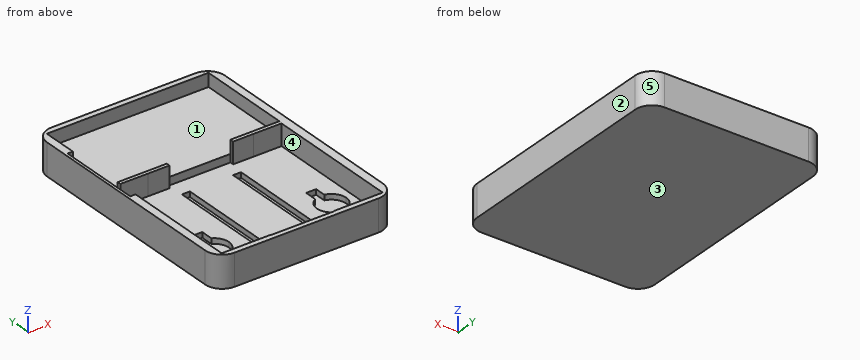
```python
from build123d import *

# Parameters (mm, degrees)
F1_DEPTH = 12
F3_DEPTH = 5
F2_W     = 24
F2_H     = 53
F5_DEPTH = 8
F6_DEPTH = 10
F7_W     = 3
F7_H     = 40
F8_DEPTH = 10
F9_DEPTH = 10


with BuildPart() as f1:
    # F0 (on Top) → F1 (new body)
    with BuildSketch(Plane.XY):
        with BuildLine():
            Line((27.15, 46.5), (-27.15, 46.5))
            ThreePointArc((-27.15, 46.5), (-31.6401280605, 44.6401280605), (-33.5, 40.15))
            Line((-33.5, 40.15), (-33.5, -40.15))
            ThreePointArc((-33.5, -40.15), (-31.6401280605, -44.6401280605), (-27.15, -46.5))
            Line((-27.15, -46.5), (27.15, -46.5))
            ThreePointArc((27.15, -46.5), (31.6401280605, -44.6401280605), (33.5, -40.15))
            Line((33.5, -40.15), (33.5, 40.15))
            ThreePointArc((33.5, 40.15), (31.6401280605, 44.6401280605), (27.15, 46.5))
        make_face()
    extrude(amount=F1_DEPTH)

    # F2 (on face) → F3 (cut)
    with BuildSketch(Plane.XY.offset(12)):
        Polygon((-30.5, 31.1559867114), (-30.5, 8.3555228412), (-12, 8.3555228412), (12, 8.3555228412), (30.5, 8.3555228412), (30.5, 44.3555228412), (-30.5, 44.3555228412), align=None)
    extrude(amount=-F3_DEPTH, mode=Mode.SUBTRACT)

    # F4 (on face) + F2 (on face) → F5 (cut)
    with BuildSketch(Plane.XY.offset(12)):
        Polygon((-19.9947099381, 7.0137236979), (-30.5000375956, 7.0301252197), (-30.5000375956, -0.696099014), (-30.5000375956, -0.6988210371), (-30.5000375956, -44.4698496722), (-12, -44.4698496722), (-12, 7.0012418968), align=None)
        with BuildLine():
            Line((-19.57828179, -19.8942141583), (-19.57828179, -24.546026914))
            ThreePointArc((-19.57828179, -24.546026914), (-17.4189463665, -26.5711645765), (-16.6222270916, -29.4223310783))
            ThreePointArc((-16.6222270916, -29.4223310783), (-25.5439247807, -33.7283715941), (-23.364767064, -24.064524212))
            Line((-23.364767064, -24.064524212), (-23.364767064, -19.8942141583))
            Line((-23.364767064, -19.8942141583), (-19.57828179, -19.8942141583))
        make_face(mode=Mode.SUBTRACT)
        Polygon((19.6427109083, 6.9518394763), (12, 6.9637717162), (12, -44.4698496722), (30.2305370569, -44.4698496722), (30.2305370569, 6.9353091531), align=None)
        with BuildLine():
            Line((23.364767064, -19.8942141583), (23.364767064, -24.064524212))
            ThreePointArc((23.364767064, -24.064524212), (26.4282676075, -26.0006333892), (27.6222270916, -29.4223310783))
            ThreePointArc((27.6222270916, -29.4223310783), (19.2710605898, -34.1256118034), (19.57828179, -24.546026914))
            Line((19.57828179, -24.546026914), (19.57828179, -19.8942141583))
            Line((19.57828179, -19.8942141583), (23.364767064, -19.8942141583))
        make_face(mode=Mode.SUBTRACT)
    with BuildSketch(Plane.XY.offset(12)):
        Polygon((-30.5, -0.696099014), (-30.5, 8.3555228412), (-30.5, 31.1559867114), (-32.5, 31.1559867114), (-32.5, -0.696099014), align=None)
        with Locations((0, -18.1444771588)):
            Rectangle(F2_W, F2_H)
        with BuildLine():
            ThreePointArc((-23.364767064, -24.064524212), (-21.4284150344, -23.9662679528), (-19.57828179, -24.546026914))
            Line((-19.57828179, -24.546026914), (-19.57828179, -19.8942141583))
            Line((-19.57828179, -19.8942141583), (-23.364767064, -19.8942141583))
            Line((-23.364767064, -19.8942141583), (-23.364767064, -24.064524212))
        make_face()
        with BuildLine():
            ThreePointArc((19.57828179, -24.546026914), (21.4284150344, -23.9662679528), (23.364767064, -24.064524212))
            Line((23.364767064, -24.064524212), (23.364767064, -19.8942141583))
            Line((23.364767064, -19.8942141583), (19.57828179, -19.8942141583))
            Line((19.57828179, -19.8942141583), (19.57828179, -24.546026914))
        make_face()
    extrude(amount=-F5_DEPTH, mode=Mode.SUBTRACT)

    # F2 (on face) → F6 (cut)
    with BuildSketch(Plane.XY.offset(12)):
        with BuildLine():
            ThreePointArc((-23.364767064, -24.064524212), (-25.5439247807, -33.7283715941), (-16.6222270916, -29.4223310783))
            ThreePointArc((-16.6222270916, -29.4223310783), (-17.4189463665, -26.5711645765), (-19.57828179, -24.546026914))
            ThreePointArc((-19.57828179, -24.546026914), (-21.4284150344, -23.9662679528), (-23.364767064, -24.064524212))
        make_face()
        with BuildLine():
            ThreePointArc((19.57828179, -24.546026914), (19.2710605898, -34.1256118034), (27.6222270916, -29.4223310783))
            ThreePointArc((27.6222270916, -29.4223310783), (26.4282676075, -26.0006333892), (23.364767064, -24.064524212))
            ThreePointArc((23.364767064, -24.064524212), (21.4284150344, -23.9662679528), (19.57828179, -24.546026914))
        make_face()
    extrude(amount=-F6_DEPTH, mode=Mode.SUBTRACT)

    # F7 (on face) → F8 (cut)
    with BuildSketch(Plane.XY.offset(12)):
        with Locations((-9.6433593556, -18.214944303)):
            Rectangle(F7_W, F7_H)
        Polygon((8.1433593556, 1.785055697), (8.1433593556, -38.214944303), (9.8566406444, -38.214944303), (11.1433593556, -38.214944303), (11.1433593556, 1.785055697), align=None)
    extrude(amount=-F8_DEPTH, mode=Mode.SUBTRACT)

    # F4 (on face) + F2 (on face) → F9 (cut)
    with BuildSketch(Plane.XY.offset(12)):
        with BuildLine():
            ThreePointArc((-16.6222270916, -29.4223310783), (-17.4189463665, -26.5711645765), (-19.57828179, -24.546026914))
            Line((-19.57828179, -24.546026914), (-19.57828179, -19.8942141583))
            Line((-19.57828179, -19.8942141583), (-23.364767064, -19.8942141583))
            Line((-23.364767064, -19.8942141583), (-23.364767064, -24.064524212))
            ThreePointArc((-23.364767064, -24.064524212), (-25.5439247807, -33.7283715941), (-16.6222270916, -29.4223310783))
        make_face()
    with BuildSketch(Plane.XY.offset(12)):
        with BuildLine():
            ThreePointArc((19.57828179, -24.546026914), (19.2710605898, -34.1256118034), (27.6222270916, -29.4223310783))
            ThreePointArc((27.6222270916, -29.4223310783), (26.4282676075, -26.0006333892), (23.364767064, -24.064524212))
            ThreePointArc((23.364767064, -24.064524212), (21.4284150344, -23.9662679528), (19.57828179, -24.546026914))
        make_face()
        with BuildLine():
            ThreePointArc((19.57828179, -24.546026914), (21.4284150344, -23.9662679528), (23.364767064, -24.064524212))
            Line((23.364767064, -24.064524212), (23.364767064, -19.8942141583))
            Line((23.364767064, -19.8942141583), (19.57828179, -19.8942141583))
            Line((19.57828179, -19.8942141583), (19.57828179, -24.546026914))
        make_face()
    extrude(amount=-F9_DEPTH, mode=Mode.SUBTRACT)


solid = f1.part
```
Could you check a few things on this model? Use its own coordinates, in mm. Face numbers are marked on the shaded views. A direction names the side the tool comes from. Round coordinates to 2 decimals unless told otherwise and drop trailing zeros. Write each loop counter-clockwise with the first axis right and the second up, starting at its lowest first coordinate (ties: lowest second). Pieces come first, ordered by that corner, then holes. Notation, with made-up numbers: M -12.75,-17 L 22.25,-17 A29 ccw 22.25,18 Z; hole C -24.75,12 d3. An arc over 180 degrees is marked long. Answer in a Markdown table with one row per item. Add a question column.
Q1. On a 3-axis mill with a long thin cutter (end or side, diameter ignored), from which of +Z, -Z, +X, -X, +Y, -Y can I reach the whole of each face in a straight line? I mean the marked faces 1 and 2. Say none if no direction works.
Q2. Imagine slicing it at C-C (y = -3). Please give me the cut outline in (x, z), then the cut area to 3 significant figures.
Q3. Imagine slicing it at A-A (z = 10). Please give me the cut outline in (x, y).
Q4. Imagine slicing it at B-B (z = 5.5). Please give me the cut outline in (x, y), then the cut area to 3 significant figures.
Q5. If we mould it in two halves opening along X, with no side actions, what happens to the marked faces 3, 4 and 5? For each: +X half, -X half, draft (parallel to the pull), parting line (faces both ways), or undercut.
Q6. If I drill on line 1 (Y direction, x = -14, z = 9); line 2 (X direction, y = -10, z = 7.25); line 3 (Y direction, x = -19.5, z = 6), over which ranges is the centre line in solid material (lowest first)? Write a range as from..to.
Q7. Will these pins go through, and if not, where does the flat tip stop? pin 1 Ø8 at (x, y) = (26, -16.5) entering from +Z; pin 2 Ø3 at (x, y) = (13.5, 7.5) entering from -Z; pin 3 Ø3 at (x, y) = (24, 36) entering from +Z; pin 4 Ø1 at (x, z) = (-31, 6.5) entering from -Y.
Q8. Imagine slicing it at D-D (x = 7). Please give me the cut outline in (y, z).
Values:
| question | item | result |
|---|---|---|
| 1 | face 1 | +Z |
| 1 | face 2 | +Z, -Z, +X, +Y, -Y |
| 2 | outline | M -33.5,0 L 33.5,0 L 33.5,12 L 30.23,12 L 30.23,4 L 11.14,4 L 11.14,2 L 8.14,2 L 8.14,4 L -8.14,4 L -8.14,2 L -11.14,2 L -11.14,4 L -30.5,4 L -30.5,12 L -33.5,12 Z |
| 2 | area | 306 mm^2 |
| 3 | outline | M -33.5,-40.15 A6.35 ccw -27.15,-46.5 L 27.15,-46.5 A6.35 ccw 33.5,-40.15 L 33.5,40.15 A6.35 ccw 27.15,46.5 L -27.15,46.5 A6.35 ccw -33.5,40.15 Z; M -30.5,7.03 L -12,7 L -12,8.36 L -30.5,8.36 Z; hole M -32.5,-0.7 L -30.5,-0.7 L -30.5,-44.47 L -12,-44.47 L -12,-44.64 L 12,-44.64 L 12,-44.47 L 30.23,-44.47 L 30.23,6.94 L 12,6.96 L 12,8.36 L 30.5,8.36 L 30.5,44.36 L -30.5,44.36 L -30.5,31.16 L -32.5,31.16 Z |
| 4 | outline | M -33.5,-40.15 A6.35 ccw -27.15,-46.5 L 27.15,-46.5 A6.35 ccw 33.5,-40.15 L 33.5,40.15 A6.35 ccw 27.15,46.5 L -27.15,46.5 A6.35 ccw -33.5,40.15 Z; hole M -32.5,-0.7 L -30.5,-0.7 L -30.5,-44.47 L -12,-44.47 L -12,-44.64 L 12,-44.64 L 12,-44.47 L 30.23,-44.47 L 30.23,6.94 L 12,6.96 L 12,8.36 L -12,8.36 L -12,7 L -30.5,7.03 L -30.5,31.16 L -32.5,31.16 Z |
| 4 | area | 2,970 mm^2 |
| 5 | face 3 | draft |
| 5 | face 4 | undercut |
| 5 | face 5 | +X half |
| 6 | line 1 | -46.5..-44.47, 7..8.36, 44.36..46.5 |
| 6 | line 2 | -33.5..-30.5, 30.23..33.5 |
| 6 | line 3 | -46.5..-44.47, 7.01..46.5 |
| 7 | pin 1 | z = 4 |
| 7 | pin 2 | z = 0 |
| 7 | pin 3 | z = 7 |
| 7 | pin 4 | y = -45.54 |
| 8 | outline | M -46.5,0 L 46.5,0 L 46.5,12 L 44.36,12 L 44.36,7 L 8.36,7 L 8.36,4 L -44.64,4 L -44.64,12 L -46.5,12 Z |
